Autodesk Inventor part; units mm, degrees
ref_plane "YZ Plane" through (0, 0, 0) normal (1, 0, 0) x (0, 1, 0)
ref_plane "XZ Plane" through (0, 0, 0) normal (0, 1, 0) x (-1, 0, 0)
ref_plane "XY Plane" through (0, 0, 0) normal (0, 0, 1) x (1, 0, 0)
sketch "Sketch1" plane through (0, 0, 0) normal (1, 0, 0) x (0, 1, 0)
  line L0 (21.25, -21) -> (-21.25, -21)
  line L1 (-21.25, -21) -> (-21.25, 21)
  line L2 (-21.25, 21) -> (21.25, 21)
  line L3 (21.25, 21) -> (21.25, -21)
  line L4 (21.25, -21) -> (-21.25, 21) construction
  line L5 (-21.25, -21) -> (21.25, 21) construction
  line L6 (-26.25, 26) -> (26.25, 26)
  line L7 (26.25, 26) -> (26.25, -26)
  line L8 (26.25, -26) -> (-26.25, -26)
  line L9 (-26.25, -26) -> (-26.25, 26)
  line L10 (-26.25, 26) -> (26.25, -26) construction
  line L11 (26.25, 26) -> (-26.25, -26) construction
  line L12 (17.25, 21) -> (21.25, 17)
  line L13 (-26.25, 0) -> (26.25, 0)
  line L14 (0, 26) -> (0, -26)
  line L15 (21.25, -21) -> (-21.25, 21) construction
  line L16 (-17.25, 21) -> (-21.25, 17)
  line L17 (21.25, -21) -> (26.25, -21)
  line L18 (-21.25, -21) -> (-26.25, -21)
  circle A0 centre (0, 0) radius 12
  line L19 (-26.25, 26) -> (26.25, 26)
  line L20 (26.25, 26) -> (26.25, 51)
  line L21 (26.25, 51) -> (-26.25, 51)
  line L22 (-26.25, 51) -> (-26.25, 26)
  point P0 (-21.25, 17)
  point P1 (-17.25, 21)
  point P2 (-21.25, 0)
  point P3 (-12, 0)
  point P4 (12, 0)
  point P5 (21.25, 0)
  dimension "d0" = 42.5
  dimension "d1" = 42
  dimension "d2" = 5
  dimension "d3" = 5
  dimension "d4" = 4
  dimension "d5" = 4
  dimension "d8" = 24
  dimension "d15" = 25
extrude "Extrusion1" add sketch "Sketch1" along normal blind 48 contours L3 L13 L7 L17 | L3 L2 L14 L6 L7 L13 | L18 L9 L13 L1 | L12 L2 L3 | L13 L9 L6 L14 L2 L1 | L6 L22 L21 L20 | L1 L2 L16
extrude "Extrusion2" add sketch "Sketch1" against normal blind 5 contours L3 L13 L7 L17 | L13 A0 L14 L2 L12 L3 | L3 L2 L14 L6 L7 L13 | L18 L9 L13 L1 | L12 L2 L3 | L13 L9 L6 L14 L2 L1 | L1 L16 L2 L14 A0 L13 | L6 L22 L21 L20 | L1 L2 L16
sketch "Sketch2" plane through (48, 0, 0) normal (1, 0, 0) x (0, 0, -1)
  line L0 (21, 26.25) -> (-51, 26.25)
  line L1 (-51, 26.25) -> (-51, -26.25)
  line L2 (-51, -26.25) -> (21, -26.25)
  line L3 (21, -26.25) -> (21, 26.25)
  point P0 (0, 0)
  point P1 (-26, -26.25)
extrude "Extrusion3" add sketch "Sketch2" along normal blind 5
sketch "Sketch4" plane through (-5, -26.25, -21) normal (0, 0, -1) x (-1, 0, 0)
  line L0 (0, 52.5) -> (0, 47.5)
  line L1 (-5, 47.5) -> (-53, 47.5)
  line L2 (0, 52.5) -> (-5, 52.5)
  line L3 (-5, 52.5) -> (-5, 47.5)
  line L4 (-5, 47.5) -> (0, 47.5)
  line L5 (0, 47.5) -> (0, 52.5)
  line L6 (0, 0) -> (0, 52.5)
  line L7 (0, 0) -> (-58, 0)
  line L8 (0, 4.8747) -> (-5, 4.8747)
  line L9 (-5, 4.8747) -> (-5, 0)
  line L10 (-5, 0) -> (0, 0)
  line L11 (0, 0) -> (0, 4.8747)
  point P0 (-5, 26.25)
extrude "Extrusion5" add sketch "Sketch4" along normal blind 25
properties part number "motor_mount"
For this review, take the finished solid that the model builds, in its own axes (mm). A direction names the side the tool comes from. Round coordinates to 2 decimals unless told otherwise and drop trailing zeros. Write each loop counter-clockwise with the first axis right and the second up, starting at its lowest first coordinate (ties: lowest second). Pieces come first, ordered by that corner, then holes.
1) Machinability: for faces 1 (the face through (21, 21.25, 0)), 2 (the face through (0, 24, -33)), 3 (the face through (-3, -21.375, -33)), 4 (the face through (-2, -17, 0)), which of the approach directions +Z, -Z, +X, -X, +Y, -Y give a long, thin tool a straight path to every point of the face, cutting with its end or side? Answer none if there is none.
Answer below:
face 1: -Z
face 2: -Z, +X, +Y, -Y
face 3: -Z, +X, -X
face 4: -Z, -X
2) Take a section at B-B on y = 0. Give the boundary of the cut face in (x, z).
Answer below:
outline: (-5, 12) - (0, 12) - (0, 21) - (48, 21) - (48, -21) - (53, -21) - (53, 51) - (-5, 51) - close
3) Take a section at D-D on z = -7. Give the boundary of the cut face in (x, y).
Answer below:
outline: (-5, -26.25) - (53, -26.25) - (53, 26.25) - (-5, 26.25) - (-5, 21.25) - (48, 21.25) - (48, -21.25) - (-5, -21.25) - close
4) Take a section at A-A on z = 14. Give the boundary of the cut face in (x, y).
Answer below:
outline: (-5, -26.25) - (53, -26.25) - (53, 26.25) - (-5, 26.25) - close; hole (0, -21.25) - (48, -21.25) - (48, 21.25) - (0, 21.25) - close
5) Mouldability with a two-part tool opening along Y and no side actions: class faces 5 (the face through (24, 26.25, 13)), 6 (the face through (24, 0, 21)), 7 (the face through (-2, -24, -46)) as +Y half, -Y half, draft (parallel to the pull), parting line (faces both ways), or undercut.
Answer below:
face 5: +Y half
face 6: undercut
face 7: draft
6) Take a section at C-C on x = 1.5. Give the boundary of the cut face in (y, z).
Answer below:
outline: (-26.25, -21) - (-21.25, -21) - (-21.25, 17) - (-17.25, 21) - (17.25, 21) - (21.25, 17) - (21.25, -21) - (26.25, -21) - (26.25, 51) - (-26.25, 51) - close
7) For line 1 along X through (y, z) = (6, 12); line 2 along Y through (x, z) = (0.5, -20); line 3 along Z through (x, y) = (21.5, 11.5), list the stretches that pass through material, from the lowest coordinate up.
Answer below:
line 1: x = -5 to 0, 48 to 53
line 2: y = -26.25 to -21.25, 21.25 to 26.25
line 3: z = 21 to 51
8) Insertion check: pin 1 Ø2.5 at (y, z) = (-23, -32) entering from +X; pin 2 Ø5.5 at (x, y) = (-3, 17) entering from -Z. Each pin has a flat end and moves straight along its axis. Give the tip position at first contact, or say it passes through.
Answer below:
pin 1: stops at x = 0
pin 2: stops at z = 0
